Design review of the part built by this model. Coordinates are the model's own, in mm. Coordinates: 2 decimals unless noted, no trailing zeros. Order: outer loops, then holes, each group sorted by start corner. A loop starts at its lowest first (then second) coordinate and runs counter-clockwise, first axis right, second up. Notation, with made-up numbers: M 49,68.25 L 62,68.25 A24 ccw 62,94.25 Z; hole C 47.5,29 d4. An arc over 180 degrees is marked long. Answer in a Markdown table with one row per item.
from build123d import *

# Parameters (mm, degrees)
F0_R     = 22.5
F1_DEPTH = 25
F2_R     = 19.5
F3_DEPTH = 20
F5_DEPTH = 25


with BuildPart() as f1:
    # F0 (on Top) → F1 (new body)
    with BuildSketch(Plane.XY):
        Circle(F0_R)
    extrude(amount=F1_DEPTH)

    # F2 (on Top) → F3 (cut)
    with BuildSketch(Plane.XY):
        Circle(F2_R)
    extrude(amount=F3_DEPTH, mode=Mode.SUBTRACT)

    # F4 (on face) → F5 (join)
    with BuildSketch(Plane(origin=(0, 0, 0), x_dir=(1, 0, 0), z_dir=(0, 0, -1))):
        with BuildLine():
            Line((-22.5, 22.5), (-22.5, 2.46e-08))
            ThreePointArc((-22.5, 2.46e-08), (-15.9099025593, 15.9099025941), (2.47e-08, 22.5))
            Line((2.47e-08, 22.5), (-22.5, 22.5))
        make_face()
        with BuildLine():
            ThreePointArc((2.47e-08, 22.5), (15.9099025854, 15.909902568), (22.5, 0))
            Line((22.5, 0), (22.5, 22.5))
            Line((22.5, 22.5), (2.47e-08, 22.5))
        make_face()
    extrude(amount=-F5_DEPTH)


solid = f1.part
(1) Draft analysis for pull direction X (two halves, no side actions). For faces 1 (the cylindrical face through (0.495, 22.495, 12.325)), 2 (the cylindrical face through (-2.539, 19.334, 9.86)), 3 (the flat face through (-22.5, -11, 12)), 4 (the flat face through (0, 0, 20)), state which applies: pulls with the +X half, pulls with the -X half, needs draft (parallel to the pull), parting line crosses it, or undercut.
Return value:
| item | result |
|---|---|
| face 1 | parting line crosses it |
| face 2 | undercut |
| face 3 | pulls with the -X half |
| face 4 | undercut |
(2) Add section B-B, the plane z = 8.25. Give the boundary of the cut face in (x, y), and give its area (3 significant figures).
Return value:
| item | result |
|---|---|
| outline | M -22.5,-22.5 L 22.5,-22.5 L 22.5,0 A22.5 ccw -22.5,0 Z; hole C 0,0 d39 |
| area | 613 mm2 |
(3) Insertion check: pin 1 Ø5 at (x, y) = (-4, 6.5) entering from -Z; pin 2 Ø10 at (x, y) = (-17, -3.5) entering from -Z; pin 3 Ø1 at (x, z) = (-13, 7) entering from +Y; pin 4 Ø2 at (y, z) = (10, 3) entering from -X. Each pin has a flat end and moves straight along its axis. Give the tip position at first contact, or say it passes through.
Return value:
| item | result |
|---|---|
| pin 1 | stops at z = 20 |
| pin 2 | stops at z = 0 |
| pin 3 | stops at y = 18.71 |
| pin 4 | stops at x = -20.62 |
(4) For line 1 along Y through (x, z) = (0, 12); line 2 along X through (y, z) = (-13, 10.5); line 3 along Y through (x, z) = (-6.5, 13.25), list the stretches that pass through material, from the lowest coordinate up. Write a range as from..to.
Return value:
| item | result |
|---|---|
| line 1 | y = -22.5..-19.5, 19.5..22.5 |
| line 2 | x = -22.5..-14.53, 14.53..22.5 |
| line 3 | y = -22.5..-18.38, 18.38..21.54 |
(5) Add section A-A, the plane x = 0. Give the boundary of the cut face in (y, z).
Return value:
| item | result |
|---|---|
| outline | M -22.5,0 L -19.5,0 L -19.5,20 L 19.5,20 L 19.5,0 L 22.5,0 L 22.5,25 L -22.5,25 Z |
(6) Add section C-C, the plane y = 17. Give the boundary of the cut face in (x, z), and give its area (3 significant figures).
Return value:
| item | result |
|---|---|
| outline | M -14.74,0 L -9.55,0 L -9.55,20 L 9.55,20 L 9.55,0 L 14.74,0 L 14.74,25 L -14.74,25 Z |
| area | 355 mm2 |
